For this review, take the finished solid that the model builds, in its own axes (mm). A direction names the side the tool comes from. Round coordinates to 2 decimals unless told otherwise and drop trailing zeros. Write each loop counter-clockwise with the first axis right and the second up, starting at its lowest first coordinate (ties: lowest second). Pieces come first, ordered by that corner, then holes.
from build123d import *

# Parameters (mm, degrees)
BOSS_EXTRUDE1_DEPTH = 100
FILLET1_R           = 50
SKETCH2_R           = 5
CUT_EXTRUDE1_DEPTH  = 116
SKETCH5_W           = 120
SKETCH5_H           = 120
BOSS_EXTRUDE4_DEPTH = 5
SKETCH6_W           = 110
SKETCH6_H           = 120
BOSS_EXTRUDE6_DEPTH = 5


with BuildPart() as part:
    # Sketch1 → Boss-Extrude1 (new body)
    with BuildSketch(Plane.XY):
        Polygon((5, -172.5), (5, -8), (5, 0), (0, 0), (0, -8), (0, -146), (0, -154), (0, -292), (0, -350), (5, -350), (5, -292), (5, -177.5), (115, -177.5), (115, -293.5), (115, -350), (120, -350), (120, -293.5), (120, -155.5), (120, -147.5), (120, -9.5), (120, 0), (115, 0), (115, -9.5), (115, -172.5), align=None)
    extrude(amount=BOSS_EXTRUDE1_DEPTH)

    # Fillet1
    fillet1_edges = [part.edges().sort_by_distance(p)[0] for p in [
        (2.5, 0, 100),
        (2.5, 0, 0),
        (117.5, -350, 0),
        (117.5, -350, 100),
        (2.5, -350, 100),
        (2.5, -350, 0),
        (117.5, 0, 100),
        (117.5, 0, 0),
    ]]
    fillet(fillet1_edges, radius=FILLET1_R - 0.0001)  # a hair under: the kernel refuses the full size

    # Sketch2 → Cut-Extrude1 (cut)
    with BuildSketch(Plane(origin=(120, 0, 0), x_dir=(0, 0, -1), z_dir=(1, 0, 0))):
        with Locations(Location((-50, -300, 0), (0, 0, 90))):
            Circle(SKETCH2_R)
        with Locations(Location((-50, -50, 0), (0, 0, 90))):
            Circle(SKETCH2_R)
    extrude(amount=-CUT_EXTRUDE1_DEPTH, mode=Mode.SUBTRACT)

    # Sketch5 → Boss-Extrude4 (add)
    with BuildSketch(Plane.XY.offset(100)):
        with Locations((60, -175)):
            Rectangle(SKETCH5_W, SKETCH5_H)
    extrude(amount=-BOSS_EXTRUDE4_DEPTH)

    # Sketch6 → Boss-Extrude6 (add)
    with BuildSketch(Plane(origin=(0, 0, 0), x_dir=(-1, 0, 0), z_dir=(0, 0, -1))):
        with Locations((-60, -175)):
            Rectangle(SKETCH6_W, SKETCH6_H)
    extrude(amount=-BOSS_EXTRUDE6_DEPTH)


solid = part.part
(1) For line 1 along Z through (x, y) = (118.1, -50); line 2 along X through (y, z) = (-247, 65); line 3 along Z through (x, y) = (55.5, -227.5), list the stretches that pass through material, from the lowest coordinate up.
Geometry check:
line 1: z = 0 to 45, 55 to 100
line 2: x = 0 to 5, 115 to 120
line 3: z = 0 to 5, 95 to 100
(2) For faces 4 (the face through (59, -173, 100)), 5 (the face through (61, -172.5, 49)), 6 (the face through (59, -177.5, 49)), 7 (the face through (4.507, -50.651, 54.957)), list the 3-axis set-ups (+Z, -Z, +X, -X, +Y, -Y) from which the entire face can be reached by the end or side of a thin tool; tool diameter is ignored.
Geometry check:
face 4: +Z, +X, -X, +Y, -Y
face 5: +Y
face 6: -Y
face 7: +X
(3) We need section D-D, the plane z = 61.5. Give the boundary of the cut face in (x, y).
Geometry check:
outline: (0, -348.66) - (5, -348.66) - (5, -177.5) - (115, -177.5) - (115, -348.66) - (120, -348.66) - (120, -1.34) - (115, -1.34) - (115, -172.5) - (5, -172.5) - (5, -1.34) - (0, -1.34) - close
(4) Mouldability with a two-part tool opening along X and no side actions: class faces 1 (the face through (5, -265, 49)), 2 (the face through (4, -300, 50)), 3 (the face through (2.535, -335.742, 84.964)) as pulls with the +X half, pulls with the -X half, needs draft (parallel to the pull), parting line crosses it, or undercut.
Geometry check:
face 1: undercut
face 2: pulls with the +X half
face 3: needs draft
(5) We need section B-B, the plane x = 75. Give the boundary of the cut face in (y, z), and give its area (3 significant figures).
Geometry check:
outline: (-235, 0) - (-115, 0) - (-115, 5) - (-172.5, 5) - (-172.5, 95) - (-115, 95) - (-115, 100) - (-235, 100) - (-235, 95) - (-177.5, 95) - (-177.5, 5) - (-235, 5) - close
area: 1,650 mm2
(6) We need section A-A, the plane y = -154.5. Give the boundary of the cut face in (x, z).
Geometry check:
outline: (0, 0) - (120, 0) - (120, 100) - (0, 100) - close; hole (5, 5) - (115, 5) - (115, 95) - (5, 95) - close
(7) For pin 1 Ø10 at (x, z) = (24.5, 20) entering from -Y; pin 2 Ø5.5 at (x, z) = (43.5, 96.5) entering from -Y; pin 3 Ø5 at (x, z) = (66.5, 21) entering from +Y, all flat-tipped, find the tip position at first contact; note any pin that passes through.
Geometry check:
pin 1: stops at y = -177.5
pin 2: stops at y = -235
pin 3: stops at y = -172.5
(8) We need section C-C, the plane y = -276.5. Give the boundary of the cut face in (x, z).
Geometry check:
outline: (0, 0) - (5, 0) - (5, 100) - (0, 100) - close; (115, 0) - (120, 0) - (120, 100) - (115, 100) - close
